Autodesk Fusion 360 part; units mm, degrees
sketch "Plate" plane through (0, 0, 0) normal (0, 1, 0) x (1, 0, 0)
  line L0 (0, 0) -> (5.4, 0)
  line L1 (5.4, 0) -> (5.4, -60)
  line L2 (5.4, -60) -> (0, -60)
  line L3 (0, -60) -> (0, 0)
  dimension "d242" = 5.4
  dimension "d243" = 60
extrude "Plate (1)" add sketch "Plate" along normal mid plane 28 from surface at -2
sketch "Hook profile" plane through (0, 0, 0) normal (0, 1, 0) x (1, 0, 0)
  line L0 (0, -58) -> (-8.3, -58)
  line L1 (-8.3, -58) -> (-8.3, -41)
  line L2 (-8.3, -41) -> (-5.3, -41)
  line L3 (-5.3, -41) -> (-3.8, -42.5)
  line L4 (-3.8, -42.5) -> (-3.8, -53)
  line L5 (-3.8, -53) -> (0, -53)
  line L6 (0, -53) -> (0, -58)
  dimension "d247" = 58
  dimension "d248" = 8.3
  dimension "d249" = 3.8
  dimension "d250" = 5
  dimension "d251" = 10.5
  dimension "d252" = 1.5
  dimension "d253" = 1.5
extrude "Hook profile (1)" add sketch "Hook profile" along normal mid plane 2.4
pattern_linear "Hook rows" count 2 spacing 25.4 along (0, 0, -1) count 3 spacing 0 along (0, 0, 1) of "Hook profile (1)"
sketch "Peg profile" plane through (0, 0, 0) normal (0, 1, 0) x (1, 0, 0)
  line L0 (5.4, -45) -> (12.2, -45)
  line L1 (12.2, -45) -> (12.2, -55.4)
  line L2 (12.2, -55.4) -> (11.6, -56)
  line L3 (11.6, -56) -> (10.2, -56)
  line L4 (10.2, -56) -> (10.2, -49)
  line L5 (10.2, -49) -> (5.4, -49)
  line L6 (5.4, -49) -> (5.4, -45)
  dimension "d260" = 5.4
  dimension "d261" = 45
  dimension "d262" = 12.2
  dimension "d263" = 55.4
  dimension "d264" = 11.6
  dimension "d265" = 56
  dimension "d266" = 10.2
  dimension "d267" = 49
extrude "Peg profile (1)" add sketch "Peg profile" along normal mid plane 4.7 from surface at -7.52
pattern_linear "Peg rows" count 2 spacing 40 along (0, 0, -1) count 3 spacing 0 along (0, 0, 1) of "Peg profile (1)"
fillet "Peg bearing fillets" radius 1.5 4 edges at (7.8, -9.87, 9) (7.8, -5.17, 9) (7.8, -9.87, 49) (7.8, -5.17, 49)
fillet "Prong front fillets" radius 1 4 edges at (12.2, -5.17, 50.2) (12.2, -5.17, 10.2) (12.2, -9.87, 10.2) (12.2, -9.87, 50.2)
equation "bracketWidth = 24.0 mm"
equation "plateThickness = 5.4 mm"
equation "plateHeight = 60.0 mm"
equation "slotWidth = 3.2 mm"
equation "slotPitchVertical = 25.4 mm"
equation "faceMetalThickness = 2.0 mm"
equation "hookTabWidth = slotWidth - 0.8 mm"
equation "hookThroat = faceMetalThickness + 1.8 mm"
equation "hookNeckHeight = 5.0 mm"
equation "hookLipThickness = 4.5 mm"
equation "hookLipDrop = 12.0 mm"
equation "hookLipChamfer = 1.5 mm"
equation "topHookNeckTop = 58.0 mm"
equation "boardThickness = 4.6 mm"
equation "boardSlotWidth = 5.0 mm"
equation "boardSlotHeight = 15.0 mm"
equation "boardPitch = 40.0 mm"
equation "pegWidth = boardSlotWidth - pegClearance"
equation "pegRootLength = boardThickness + pegRootProud"
equation "pegRootHeight = 4.0 mm"
equation "pegProngThickness = 2.0 mm"
equation "pegTotalHeight = boardSlotHeight - 4 mm"
equation "pegProngChamfer = 0.6 mm"
equation "pegBearingFillet = 1.5 mm"
equation "topPegRootZ = 45.0 mm"
equation "pegOffsetY = -7.52 mm"
equation "plateInboardExtension = 4.0 mm"
equation "pegClearance = 0.3 mm"
equation "pegRootProud = 0.2 mm"
equation "pegProngFrontFillet = 1.0 mm"
equation "d242 = plateThickness"
equation "d243 = plateHeight"
equation "d244 = -plateInboardExtension / 2"
equation "d245 = bracketWidth + plateInboardExtension"
equation "d247 = topHookNeckTop"
equation "d248 = hookThroat + hookLipThickness"
equation "d249 = hookThroat"
equation "d250 = hookNeckHeight"
equation "d251 = hookLipDrop - hookLipChamfer"
equation "d252 = hookLipChamfer"
equation "d253 = hookLipChamfer"
equation "d254 = hookTabWidth"
equation "d260 = plateThickness"
equation "d261 = topPegRootZ"
equation "d262 = plateThickness + pegRootLength + pegProngThickness"
equation "d263 = topPegRootZ + pegTotalHeight - pegProngChamfer"
equation "d264 = plateThickness + pegRootLength + pegProngThickness - pegProngChamfer"
equation "d265 = topPegRootZ + pegTotalHeight"
equation "d266 = plateThickness + pegRootLength"
equation "d267 = topPegRootZ + pegRootHeight"
equation "d268 = pegOffsetY"
equation "d269 = pegWidth"
equation "d276 = pegBearingFillet"
equation "d278 = pegProngFrontFillet"
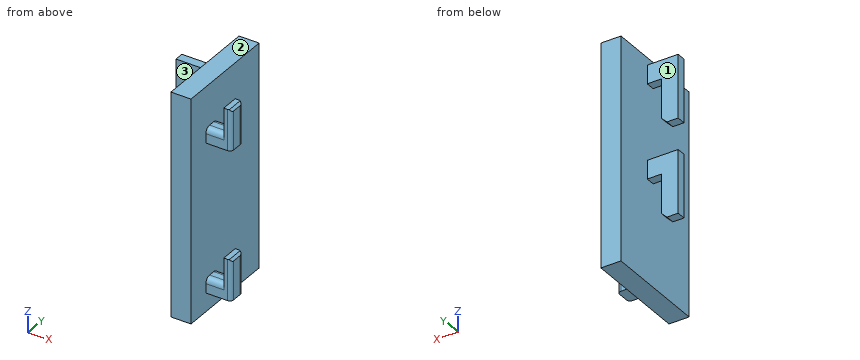
Read the model definition and answer for the solid it produces. Units are mm, in the model's axes. Face numbers are marked on the shaded views. A direction names the side the tool comes from. Round coordinates to 2 decimals unless told otherwise and drop trailing zeros. Order: outer loops, then holes, each group sorted by start corner. A loop starts at its lowest first (then second) coordinate and runs counter-clockwise, first axis right, second up.
1) Straight lines are drawn through the part: L1, parallel to X at y = 2.75, z = 43.5; L2, parallel to Y at x = -6.5, z = 45; L3, parallel to X at y = -6.5, z = 47. For each, find the intervals that lie inside material, in ascending order.
2) For the marked faces 1, 2 and 3, determine the directions among +Z, -Z, +X, -X, +Y, -Y from which every point of the face is accessible in a straight line to the end or side of a thin tool.
3) Flat-ended cylindrical pins translate along their axes: pin 1 (2 mm diameter, centred on x = -4, y = 4, fed in from -Z); pin 2 (2.5 mm diameter, centred on x = -2.5, y = 0.5, fed in from -Z); pin 3 (1.2 mm diameter, centred on x = -5, y = 0, fed in from +Z); pin 4 (1.1 mm diameter, centred on x = 10.5, y = -7.5, fed in from +Z). Find the tip coordinate at first contact, or state that the pin passes through.
4) The part is cut by section B-B on z = 19.5. Write down the section's boundary in (x, y), plus the area to 3 significant figures.
5) The part is cut by section C-C on x = -1. Write down the section's boundary in (y, z), plus the area to 3 significant figures.
6) The part is cut by section A-A on x = 7.5. Write down the section's boundary in (y, z), plus the area to 3 significant figures.
7) The part is cut by section D-D on y = -2.5. Write down the section's boundary in (x, z), plus the area to 3 significant figures.
Resolved:
1. L1: x = 0 to 5.4
1. L2: y = -1.2 to 1.2
1. L3: x = 0 to 12.2
2. face 1: +Z, -Z, -X, +Y
2. face 2: +Z, +X, -X, +Y, -Y
2. face 3: +Z, -Z, -X, -Y
3. pin 1: passes through
3. pin 2: stops at z = 27.6
3. pin 3: stops at z = 58
3. pin 4: stops at z = 56
4. outline: (-8.3, -1.2) - (-3.8, -1.2) - (-3.8, 1.2) - (-8.3, 1.2) - close; (0, -16) - (5.4, -16) - (5.4, 12) - (0, 12) - close
4. area: 162 mm2
5. outline: (-1.2, 27.6) - (1.2, 27.6) - (1.2, 32.6) - (-1.2, 32.6) - close; (-1.2, 53) - (1.2, 53) - (1.2, 58) - (-1.2, 58) - close
5. area: 24.0 mm2
6. outline: (-9.87, 5) - (-5.17, 5) - (-5.17, 7.5) arc R1.5 ccw to (-6.67, 9) - (-8.37, 9) arc R1.5 ccw to (-9.87, 7.5) - close; (-9.87, 45) - (-5.17, 45) - (-5.17, 47.5) arc R1.5 ccw to (-6.67, 49) - (-8.37, 49) arc R1.5 ccw to (-9.87, 47.5) - close
6. area: 35.7 mm2
7. outline: (0, 0) - (5.4, 0) - (5.4, 60) - (0, 60) - close
7. area: 324 mm2
